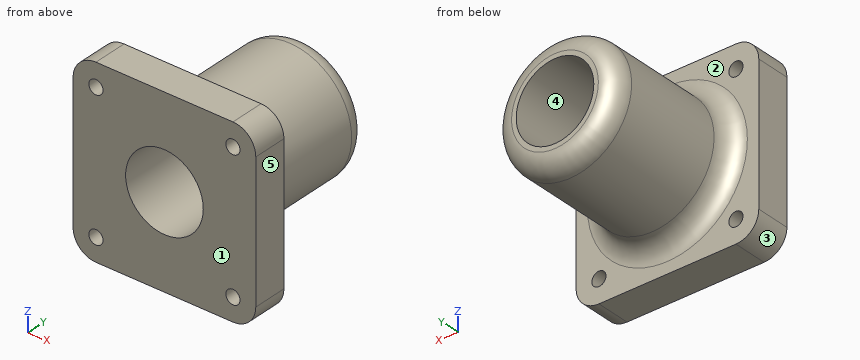
Autodesk Fusion 360 part; units mm, degrees
sketch "Sketch1" plane through (0, 0, 0) normal (0, 1, 0) x (1, 0, 0)
  line L0 (15, 20) -> (-15, 20)
  line L1 (-20, 15) -> (-20, -15)
  line L2 (-15, -20) -> (15, -20)
  line L3 (20, -15) -> (20, 15)
  line L4 (20, 20) -> (-20, -20) construction
  line L5 (-20, 20) -> (20, -20) construction
  arc A0 (20, 15) -> (15, 20) centre (15, 15) ccw
  arc A1 (-20, -15) -> (-15, -20) centre (-15, -15) ccw
  arc A2 (15, -20) -> (20, -15) centre (15, -15) ccw
  arc A3 (-15, 20) -> (-20, 15) centre (-15, 15) ccw
  circle A4 centre (-15, 15) radius 1.55
  circle A5 centre (15, 15) radius 1.55
  circle A6 centre (15, -15) radius 1.55
  circle A7 centre (-15, -15) radius 1.55
  circle A8 centre (0, 0) radius 8.5
  dimension "d1" = 40
  dimension "d2" = 5
  dimension "d4" = 3.1
  dimension "d5" = 17
extrude "Extrude1" add sketch "Sketch1" along normal blind 7.5
sketch "Sketch2" plane through (0, 7.5, 0) normal (0, 1, 0) x (-1, 0, 0)
  circle A0 centre (15, -15) radius 1.55
  circle A1 centre (-15, -15) radius 1.55
  circle A2 centre (-15, 15) radius 1.55
  circle A3 centre (15, 15) radius 1.55
  circle A4 centre (0, 0) radius 8.5
  arc A5 (15, -20) -> (20, -15) centre (15, -15) ccw
  line L0 (20, -15) -> (20, 15)
  arc A6 (20, 15) -> (15, 20) centre (15, 15) ccw
  line L1 (15, 20) -> (-15, 20)
  arc A7 (-15, 20) -> (-20, 15) centre (-15, 15) ccw
  line L2 (-20, 15) -> (-20, -15)
  arc A8 (-20, -15) -> (-15, -20) centre (-15, -15) ccw
  line L3 (-15, -20) -> (15, -20)
  circle A9 centre (0, 0) radius 8.5
  circle A10 centre (0, 0) radius 13.5
  dimension "d8" = 5
extrude "Extrude2" add sketch "Sketch2" along normal blind 30 contours A10
fillet "Fillet1" radius 4 1 faces at (-13.4329, 27.5, -1.3442)
sketch "Sketch3" plane through (0, 7.5, 0) normal (0, 1, 0) x (-1, 0, 0)
  arc A0 (15, -20) -> (20, -15) centre (15, -15) ccw
  line L0 (20, -15) -> (20, 15)
  arc A1 (20, 15) -> (15, 20) centre (15, 15) ccw
  line L1 (15, 20) -> (-15, 20)
  arc A2 (-15, 20) -> (-20, 15) centre (-15, 15) ccw
  line L2 (-20, 15) -> (-20, -15)
  arc A3 (-20, -15) -> (-15, -20) centre (-15, -15) ccw
  line L3 (-15, -20) -> (15, -20)
  circle A4 centre (15, 15) radius 1.55
  circle A5 centre (-15, -15) radius 1.55
  circle A6 centre (15, -15) radius 1.55
  circle A7 centre (-15, 15) radius 1.55
  circle A8 centre (0, 0) radius 17.5
Build history of the part. All positions in model axes, mm. Face numbers are marked on the shaded views. A direction names the side the tool comes from. Round coordinates to 2 decimals unless told otherwise and drop trailing zeros. Order: outer loops, then holes, each group sorted by start corner. A loop starts at its lowest first (then second) coordinate and runs counter-clockwise, first axis right, second up. Notation, with made-up numbers: (-32, 35.5) - (-25, 35.5) arc R32 ccw to (-25, 64.5) - close; hole circle Ø5 at (-35.5, -14). An arc over 180 degrees is marked (long way). Use a Markdown table: item, result.
1) Saw through at A-A on y = 22. Write the cut outline in (x, z).
Recorded:
| item | result |
|---|---|
| outline | circle Ø27 at (0, 0); hole circle Ø17 at (0, 0) |
2) Flat gauge pins, fed straight in: pin 1 Ø1 at (x, y) = (-3.5, 9.5) entering from +Z; pin 2 Ø4 at (x, z) = (15, -15) entering from -Y; pin 3 Ø10 at (x, y) = (13, 14.5) entering from -Z; pin 4 Ø1 at (y, z) = (22, -11) entering from +X. Where does each tip first touch, or does it go through?
Recorded:
| item | result |
|---|---|
| pin 1 | stops at z = 13.96 |
| pin 2 | stops at y = 0 |
| pin 3 | stops at z = -10.87 |
| pin 4 | stops at x = 8.49 |
3) Wall check: L1, parallel to X at y = 5.5, z = 15; L2, parallel to Z at x = 0, y = 26; L3, parallel to Y at x = 17, z = -13.5. Give the ranges that are in metal, low to high.
Recorded:
| item | result |
|---|---|
| L1 | x = -20 to -16.55, -13.45 to 13.45, 16.55 to 20 |
| L2 | z = -13.5 to -8.5, 8.5 to 13.5 |
| L3 | y = 0 to 7.5 |
4) Pull direction Z, two halves, no side cores. Call the marked faces 3, 4 and 5: pulls with the +Z half, pulls with the -Z half, needs draft (parallel to the pull), parting line crosses it, or undercut.
Recorded:
| item | result |
|---|---|
| face 3 | pulls with the -Z half |
| face 4 | undercut |
| face 5 | needs draft |
5) Tool access for the marked faces 1 and 2: list every direction of +Z, -Z, +X, -X, +Y, -Y with a clear straight run to the whole face (end or side of a thin tool).
Recorded:
| item | result |
|---|---|
| face 1 | +Z, -Z, +X, -X, -Y |
| face 2 | +Y |
